from build123d import *

# Parameters (mm, degrees)
F0_R             = 1.7859375
F0_R_2           = 7.9375
F1_DEPTH         = 9.525
F2_W             = 9.5377
F2_H             = 31.75
F3_DEPTH         = 1.5875
F5_D             = 3.571875
F5_DEPTH         = 19.05
F5_TIP           = 1.0730995118
F7_D             = 3.571875
F7_DEPTH         = 19.05
F7_TIP           = 1.0730995118
F11_D            = 3.571875
F11_DEPTH        = 12.7
F11_TIP          = 1.0730995118
F11_ON_F9_D      = 3.571875
F11_ON_F9_DEPTH  = 12.7
F11_ON_F9_TIP    = 1.0730995118
F11_ON_F10_D     = 3.571875
F11_ON_F10_DEPTH = 12.7
F11_ON_F10_TIP   = 1.0730995118


# Not quite as in the source:
# - a feature names something its author has since deleted; it is built from what else it names


with BuildPart() as f1:
    # F0 (on Front) → F1 (new body)
    with BuildSketch(Plane.XZ):
        with BuildLine():
            Line((0, 50.8), (0, 0))
            Line((0, 0), (295.275, 0))
            Line((295.275, 0), (295.275, 50.8))
            Line((295.275, 50.8), (107.9627, 50.8))
            Line((107.9627, 50.8), (107.9627, 38.1))
            ThreePointArc((107.9627, 38.1), (111.1377, 34.925), (107.9627, 31.75))
            Line((107.9627, 31.75), (98.425, 31.75))
            ThreePointArc((98.425, 31.75), (95.25, 34.925), (98.425, 38.1))
            Line((98.425, 38.1), (98.425, 50.8))
            Line((98.425, 50.8), (85.725, 50.8))
            Line((85.725, 50.8), (85.725, 23.8125))
            ThreePointArc((85.725, 23.8125), (79.375, 17.4625), (73.025, 23.8125))
            Line((73.025, 23.8125), (73.025, 50.8))
            Line((73.025, 50.8), (0, 50.8))
        make_face()
        with Locations((227.17125, 25.4)):
            Circle(F0_R, mode=Mode.SUBTRACT)
        with Locations((247.015, 25.4)):
            Circle(F0_R_2, mode=Mode.SUBTRACT)
        with Locations((266.85875, 25.4)):
            Circle(F0_R, mode=Mode.SUBTRACT)
    extrude(amount=F1_DEPTH)

    # F2 (on face) → F3 (cut)
    with BuildSketch(Plane(origin=(0, 0, 0), x_dir=(-1, 0, 0), z_dir=(0, 1, 0))):
        with Locations((-103.19385, 15.875)):
            Rectangle(F2_W, F2_H)
    extrude(amount=-F3_DEPTH, mode=Mode.SUBTRACT)

    # F5
    with Locations(Plane(origin=(0, 0, 0), x_dir=(0, -1, 0), z_dir=(-1, 0, 0))):
        with Locations((4.7625, 38.1), (4.7625, 25.4), (4.7625, 12.7)):
            Hole(F5_D / 2, depth=F5_DEPTH)
            with Locations((0, 0, -(F5_DEPTH + F5_TIP / 2))):  # 118° drill point
                Cone(0, F5_D / 2, F5_TIP, mode=Mode.SUBTRACT)

    # F7
    with Locations(Plane.XY.offset(31.75)):
        with Locations((103.19385, -5.55625)):
            Hole(F7_D / 2, depth=F7_DEPTH)
            with Locations((0, 0, -(F7_DEPTH + F7_TIP / 2))):  # 118° drill point
                Cone(0, F7_D / 2, F7_TIP, mode=Mode.SUBTRACT)

    # F11
    with Locations(Plane.XY.offset(50.8)):
        with Locations((257.175, -4.7625)):
            Hole(F11_D / 2, depth=F11_DEPTH)
            with Locations((0, 0, -(F11_DEPTH + F11_TIP / 2))):  # 118° drill point
                Cone(0, F11_D / 2, F11_TIP, mode=Mode.SUBTRACT)

    # F11 on F9
    with Locations(Plane.XY.offset(50.8)):
        with Locations((38.1, -4.7625)):
            Hole(F11_ON_F9_D / 2, depth=F11_ON_F9_DEPTH)
            with Locations((0, 0, -(F11_ON_F9_DEPTH + F11_ON_F9_TIP / 2))):  # 118° drill point
                Cone(0, F11_ON_F9_D / 2, F11_ON_F9_TIP, mode=Mode.SUBTRACT)

    # F11 on F10
    with Locations(Plane(origin=(0, 0, 0), x_dir=(1, 0, 0), z_dir=(0, 0, -1))):
        with Locations((38.1, 4.7625), (257.175, 4.7625)):
            Hole(F11_ON_F10_D / 2, depth=F11_ON_F10_DEPTH)
            with Locations((0, 0, -(F11_ON_F10_DEPTH + F11_ON_F10_TIP / 2))):  # 118° drill point
                Cone(0, F11_ON_F10_D / 2, F11_ON_F10_TIP, mode=Mode.SUBTRACT)


solid = f1.part
Read the model definition and answer for the solid it produces. Units are mm, in the model's axes. A direction names the side the tool comes from. Coordinates: 2 decimals unless noted, no trailing zeros. Write item = value, one per line. Start each with the question number.
1) Find the intervals of material crossed by L1, parallel to X at y = -2.75, z = 45 (3 decimals); L2, parallel to X at y = -4.75, z = 13.5 (3 decimals); L3, parallel to Y at x = 9.75, z = 12.7 (3 decimals), in increasing order. Write a range as from..to.
2) The mould has two halves that part along X. Classify faces 4 (the face through (37, -7, 50.8)), 5 (the face through (111.137, -4.696, 34.995)), 6 (the face through (0, -7, 26)): pulls with the +X half, pulls with the -X half, needs draft (parallel to the pull), parting line crosses it, or undercut.
3) For faces 1 (the face through (103, -1.588, 16)), 2 (the face through (107.963, -5, 45)), 3 (the face through (95.25, -4.7, 34.86)), determine the directions among +Z, -Z, +X, -X, +Y, -Y from which every point of the face is accessible in a straight line to the end or side of a thin tool.
4) Given P1, Ø2.5, axis at x = 103.5, y = -7.5, coming from the +Z side; P2, Ø5, axis at x = 237, y = -6.5, coming from the -Z side; P3, Ø2, axis at x = 38.1, y = -4.76, coming from the +Z side; P4, Ø3, axis at y = -4.76, z = 12.7, coming from the -X side, each flat-ended and moving along its own axis, determine where each tip first touches the part or whether it passes through.
Result:
q1.L1 = 0..73.025, 85.725..98.425, 107.963..295.275
q1.L2 = 19.642..37.646, 38.554..101.6, 104.787..256.721, 257.629..295.275
q1.L3 = -9.525..-6.548, -2.977..0
q2.face_4 = needs draft
q2.face_5 = undercut
q2.face_6 = pulls with the -X half
q3.face_1 = +Z, -Z, +Y
q3.face_2 = +Z, +Y, -Y
q3.face_3 = +Y, -Y
q4.P1 = 31.75
q4.P2 = 0
q4.P3 = 37.63
q4.P4 = 19.22
